Geometry check sheet. Reference: drawing and pictorial views, mm from the part's lowest x, y, z. Coordinates: 2 decimals unless noted, no trailing zeros. Loops run counter-clockwise (first coordinate to the right, second up) from the corner with the lowest first, then second, coordinate; pieces in that order, holes last. Notation, with made-up numbers: (69.25, 13) -> (99.25, 13) arc R13 ccw to (99.25, 29) -> close; hole circle Ø2 at (61.5, 17.25). An arc over 180 degrees is marked (long way). Answer as a JSON object with one key per item and string values. Group by question number.
Q1. Scan lines: L1, parallel to Y at x = 22, z = 2.75 (1 decimal); L2, parallel to X at y = 22.5, z = 0.65; L3, parallel to Y at x = 18, z = 2 (1 decimal). Record each from-to range of solid material in increasing order.
Q2. Gauge pin test, flat ends, axial feed: pin 1 Ø1 at (y, z) = (32.5, 1.5) entering from -X; pin 2 Ø8 at (x, y) = (23.47, 7.94) entering from +Z (1 decimal). Record the tip position at first contact, or that the pin passes through.
Q3. Release check for a two-part mould opening along X. For the marked faces 1 and 2 record: released by +X, released by -X, zero draft, split by the parting line, or undercut.
Q4. Cross-section at B-B on x = 25. Record the boundary of the cut face in (y, z) (1 decimal), and give its area (3 significant figures).
Q5. Cross-section at D-D on x = 6.5. Record the boundary of the cut face in (y, z) (1 decimal).
Q6. Cross-section at C-C on z = 0.65. Record the boundary of the cut face in (x, y) (1 decimal), and give its area (3 significant figures).
Q7. Cross-section at A-A on y = 32.5. Record the boundary of the cut face in (x, z) (1 decimal).
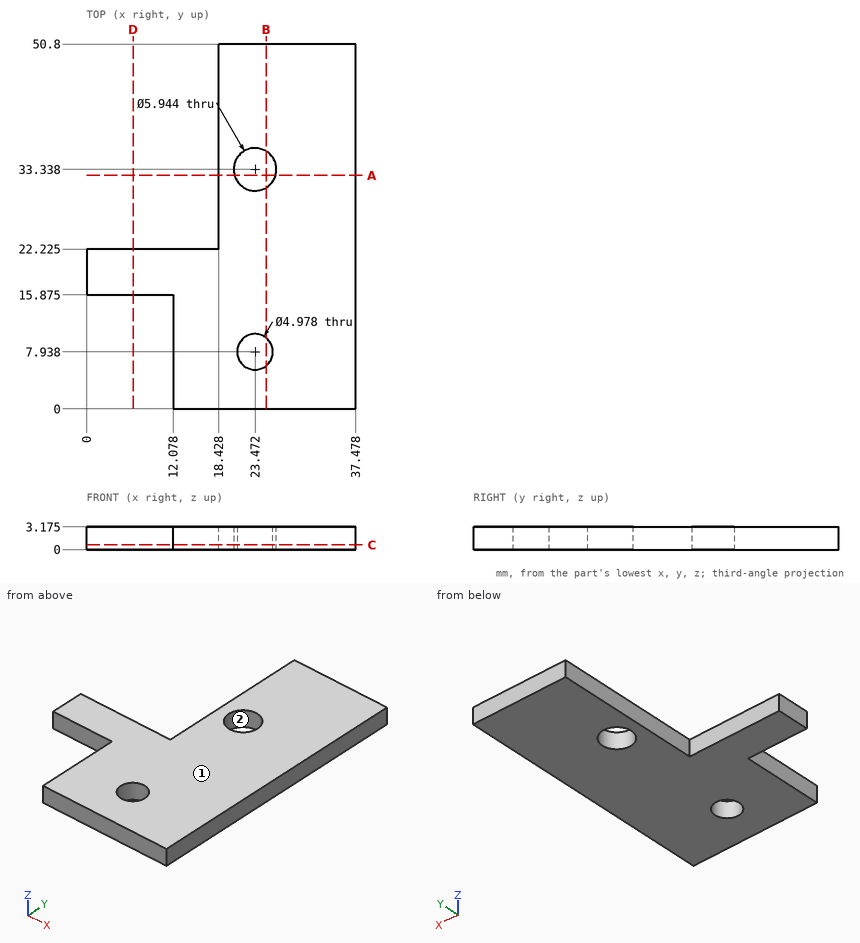
Computed values:
{
 "1": {"L1": "y = 0 to 5.9, 9.9 to 30.8, 35.9 to 50.8", "L2": "x = 18.43 to 37.48", "L3": "y = 0 to 22.2"},
 "2": {"pin 1": "stops at x = 18.43", "pin 2": "stops at z = 3.2"},
 "3": {"face 1": "zero draft", "face 2": "undercut"},
 "4": {"outline": "(0, 0) -> (6, 0) -> (6, 3.2) -> (0, 3.2) -> close; (9.9, 0) -> (30.8, 0) -> (30.8, 3.2) -> (9.9, 3.2) -> close; (35.9, 0) -> (50.8, 0) -> (50.8, 3.2) -> (35.9, 3.2) -> close", "area": "133 mm²"},
 "5": {"outline": "(15.9, 0) -> (22.2, 0) -> (22.2, 3.2) -> (15.9, 3.2) -> close"},
 "6": {"outline": "(0, 15.9) -> (12.1, 15.9) -> (12.1, 0) -> (37.5, 0) -> (37.5, 50.8) -> (18.4, 50.8) -> (18.4, 22.2) -> (0, 22.2) -> close; hole circle Ø5.9 at (23.5, 33.3); hole circle Ø5 at (23.5, 7.9)", "area": "1,140 mm²"},
 "7": {"outline": "(18.4, 0) -> (20.6, 0) -> (20.6, 3.2) -> (18.4, 3.2) -> close; (26.3, 0) -> (37.5, 0) -> (37.5, 3.2) -> (26.3, 3.2) -> close"}
}
